Geometry check sheet. Reference: the model listing, model coordinates, mm. A direction names the side the tool comes from. Round coordinates to 2 decimals unless told otherwise and drop trailing zeros. Order: outer loops, then holes, each group sorted by start corner. A loop starts at its lowest first (then second) coordinate and runs counter-clockwise, first axis right, second up.
(1) Sectioned sample at A-A (x = 1.5). Record the boundary of the cut face in (y, z).
(2) Sectioned sample at C-C (y = 3.45). Record the boundary of the cut face in (x, z).
(3) Set-up check for faces 1 (the face through (-2, 1, -4.456)), 2 (the face through (3.11, 3, 2)), 3 (the face through (-2, 3, 6.344)), 4 (the face through (-2, 3, -3.456)), 5 (the face through (-6.69, 3, 2)): record each of +Z, -Z, +X, -X, +Y, -Y from which the full face is reachable in a straight line by a thin tool's end or side.
(4) Sectioned sample at D-D (z = 6.5). Record the boundary of the cut face in (x, y).
(5) Material ranges on line 1 along X through (y, z) = (4.6, 3.75); line 2 along Z through (x, y) = (1.5, 4.35); line 3 along Y through (x, z) = (2.5, 6.5), recorded low to high.
(6) Sectioned sample at B-B (z = 3.5). Record the boundary of the cut face in (x, y), plus the area to 3 significant figures.
(7) Go/stop test with flat-tipped pins: pin 1 (0.9 mm diameter, centred on x = 0.5, y = 4, fed in from +Z); pin 2 (0.9 mm diameter, centred on x = 0, y = 4, fed in from -Z); pin 3 (2 mm diameter, centred on y = 3.5, z = 1, fed in from +X). Record where each tip stops, or that it passes through.
from build123d import *

# Parameters (mm, degrees)
SKETCH1_W           = 9.8
SKETCH1_H           = 9.8
BOSS_EXTRUDE4_DEPTH = 5
SKETCH1_4_W         = 11.8
SKETCH1_4_H         = 11.8
SKETCH1_4_W_2       = 9.8
SKETCH1_4_H_2       = 9.8
BOSS_EXTRUDE5_DEPTH = 2


with BuildPart() as part:
    # Sketch1 → Boss-Extrude4 (new body)
    with BuildSketch(Plane(origin=(0, 0, 0), x_dir=(1, 0, 0), z_dir=(0, 1, 0))):
        with Locations((-1.789763059, -1.443740832)):
            Rectangle(SKETCH1_W, SKETCH1_H)
    extrude(amount=BOSS_EXTRUDE4_DEPTH)

    # Sketch1<4> → Boss-Extrude5 (add)
    with BuildSketch(Plane(origin=(0, 0, 0), x_dir=(1, 0, 0), z_dir=(0, 1, 0))):
        with Locations((-1.789763059, -1.443740832)):
            Rectangle(SKETCH1_4_W, SKETCH1_4_H)
        with Locations((-1.789763059, -1.443740832)):
            Rectangle(SKETCH1_4_W_2, SKETCH1_4_H_2, mode=Mode.SUBTRACT)
    extrude(amount=BOSS_EXTRUDE5_DEPTH)


solid = part.part
Answer below:
1. outline: (0, -4.46) - (2, -4.46) - (2, -3.46) - (5, -3.46) - (5, 6.34) - (2, 6.34) - (2, 7.34) - (0, 7.34) - close
2. outline: (-6.69, -3.46) - (3.11, -3.46) - (3.11, 6.34) - (-6.69, 6.34) - close
3. face 1: -Z, +X, -X, +Y, -Y
3. face 2: +Z, -Z, +X, +Y
3. face 3: +Z, +X, -X, +Y
3. face 4: -Z, +X, -X, +Y
3. face 5: +Z, -Z, -X, +Y
4. outline: (-7.69, 0) - (4.11, 0) - (4.11, 2) - (-7.69, 2) - close
5. line 1: x = -6.69 to 3.11
5. line 2: z = -3.46 to 6.34
5. line 3: y = 0 to 2
6. outline: (-7.69, 0) - (4.11, 0) - (4.11, 2) - (3.11, 2) - (3.11, 5) - (-6.69, 5) - (-6.69, 2) - (-7.69, 2) - close
6. area: 53.0 mm2
7. pin 1: stops at z = 6.34
7. pin 2: stops at z = -3.46
7. pin 3: stops at x = 3.11
